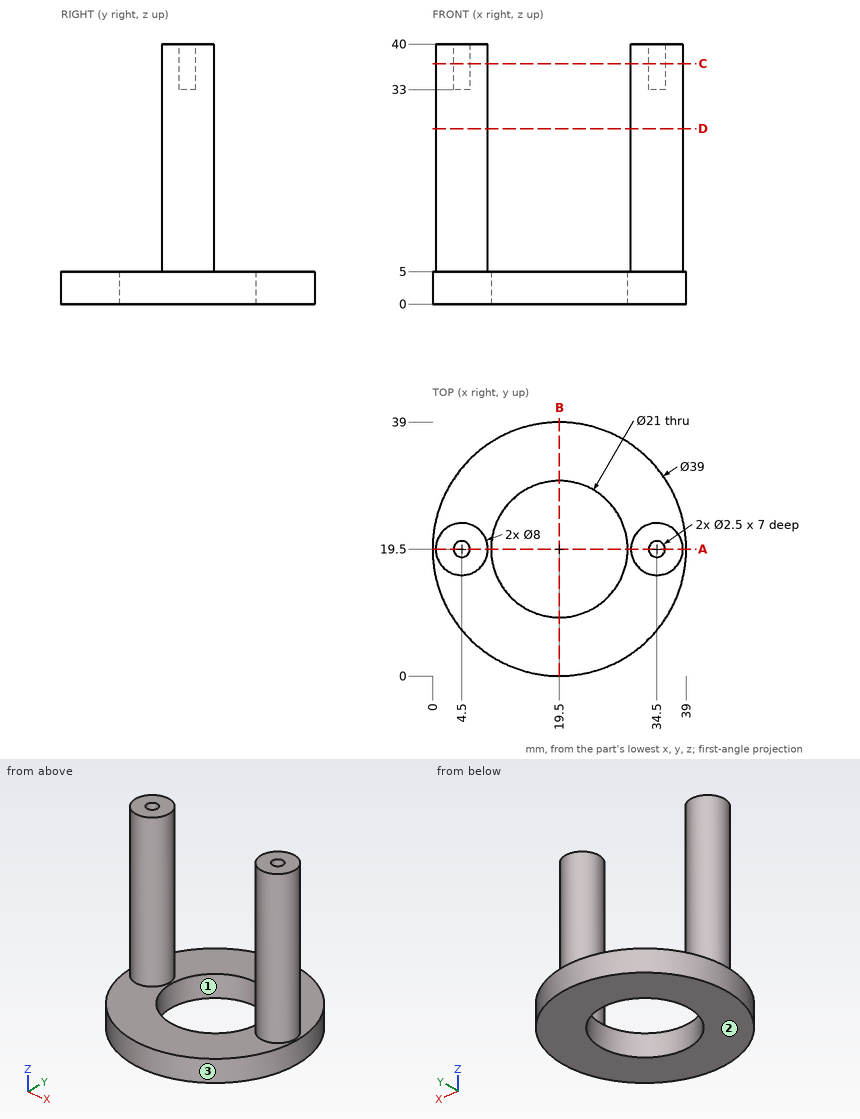
Here's the drawing with two shaded views (mm, measured from the low corner). I have some questions. Coordinates: 2 decimals unless noted, no trailing zeros. Loops run counter-clockwise (first coordinate to the right, second up) from the corner with the lowest first, then second, coordinate; pieces in that order, holes last. Notation, with made-up numbers: M 57.5,23.25 L 65.5,23.25 A13 cw 65.5,48.25 Z; hole C 84.25,-37.5 d7. An arc over 180 degrees is marked long. Put each result on its own line as item: value. Start each with the question number.
(1) Will these pins go through, and if not, where does the flat tip stop? pin 1 Ø4 at (y, z) = (17.5, 19) entering from -X; pin 2 Ø0.8 at (x, y) = (4, 19.5) entering from +Z; pin 3 Ø5 at (x, y) = (22.5, 31.5) entering from +Z; pin 4 Ø12 at (y, z) = (34, 14) entering from -X.
(2) We'd pull the mould along Y, two halves only. Please class the marked faces 1, 2 and 3: +Y half, -Y half, draft (parallel to the pull), parting line (faces both ways), or undercut.
(3) Imagine slicing it at D-D on z = 27. List the corners of the cut face in (x, y) for me, and give its area (3 significant figures).
(4) Imagine slicing it at A-A on y = 19.5. List the corners of the cut face in (x, z) for me, and give its area (3 significant figures).
(5) I need wall thicknesses on probe 1 along X at (y, z) = (19, 34); probe 2 along Y at (x, z) = (4.5, 35.25); probe 3 along Z at (x, y) = (14, 33.5). Which ranges of each line are inside material? Lowest first, please.
(6) Imagine slicing it at C-C on z = 37. List the corners of the cut face in (x, y) for me.
(7) Imagine slicing it at B-B on x = 19.5. List the corners of the cut face in (y, z) for me, and give its area (3 significant figures).
Worked answers:
1. pin 1: stops at x = 0.5
1. pin 2: stops at z = 33
1. pin 3: stops at z = 5
1. pin 4: passes through
2. face 1: undercut
2. face 2: draft
2. face 3: parting line
3. outline: C 4.5,19.5 d8; C 34.5,19.5 d8
3. area: 101 mm2
4. outline: M 0,0 L 9,0 L 9,5 L 8.5,5 L 8.5,40 L 5.75,40 L 5.75,33 L 3.25,33 L 3.25,40 L 0.5,40 L 0.5,5 L 0,5 Z; M 30,0 L 39,0 L 39,5 L 38.5,5 L 38.5,40 L 35.75,40 L 35.75,33 L 33.25,33 L 33.25,40 L 30.5,40 L 30.5,5 L 30,5 Z
4. area: 615 mm2
5. probe 1: x = 0.53 to 3.35, 5.65 to 8.47, 30.53 to 33.35, 35.65 to 38.47
5. probe 2: y = 15.5 to 18.25, 20.75 to 23.5
5. probe 3: z = 0 to 5
6. outline: C 4.5,19.5 d8; C 34.5,19.5 d8; hole C 4.5,19.5 d2.5; hole C 34.5,19.5 d2.5
7. outline: M 0,0 L 9,0 L 9,5 L 0,5 Z; M 30,0 L 39,0 L 39,5 L 30,5 Z
7. area: 90.0 mm2
